from build123d import *


with BuildPart() as f1:
    # F0 (on Front) → F1 (revolve)
    with BuildSketch(Plane.XZ):
        Polygon((0, 8), (0, 0), (4, 0), (4, 8.25), (4, 9), (0, 9), align=None)
        Polygon((4, 9), (4, 8.25), (6, 8.25), (6, 11), (4, 11), align=None)
    revolve(axis=Axis((0, 0, 4), (0, 0, 1)))


solid = f1.part
Check sheet for the modelled part. Datum: model origin and axes. Units: mm. A direction names the side the tool comes from. Round coordinates to 2 decimals unless told otherwise and drop trailing zeros. Order: outer loops, then holes, each group sorted by start corner. A loop starts at its lowest first (then second) coordinate and runs counter-clockwise, first axis right, second up.
(1) Access from +Z, -Z, +X, -X, +Y, -Y to the whole of each face (thin tool, end or side, straight path). Record for faces 1 (the flat face through (0, 0, 0)), 2 (the flat face through (1.42, -3.92, 8.25)), 3 (the flat face through (0, 0, 9)).
(2) Go/stop test with flat-tipped pins: P1, Ø2, axis at x = 0, z = 4, coming from the +Y side; P2, Ø3, axis at y = -4.5, z = 5.5, coming from the +X side; P3, Ø2.5, axis at x = 0, y = -1, coming from the +Z side. Record where each tip stops, or that it passes through.
(3) Scan lines: probe 1 along Y at (x, z) = (0, 10.15); probe 2 along Z at (x, y) = (-1.75, 5.5); probe 3 along Z at (x, y) = (1.25, 1.75). Record each from-to range of solid material in increasing order.
(4) Cross-section at C-C, the plane z = 9.75. Enter the section's corners in (x, y).
(5) Cross-section at A-A, the plane x = 0. Enter the section's corners in (y, z), and give its area (3 significant figures).
(6) Cross-section at D-D, the plane z = 5. Enter the section's corners in (x, y), and give its area (3 significant figures).
(7) Draft check along Y on faces 4 (the flat face through (-1.42, -3.92, 11)), 5 (the cylindrical face through (-0.867, -3.905, 4.183)), 6 (the cylindrical face through (-0.867, -3.905, 9.986)). Enter one of: pulls with the +Y half, pulls with the -Y half, needs draft (parallel to the pull), parting line crosses it, or undercut.
Check sheet entries:
1. face 1: -Z, +X, -X, +Y, -Y
1. face 2: -Z
1. face 3: +Z
2. P1: stops at y = 4
2. P2: stops at x = 2.65
2. P3: stops at z = 9
3. probe 1: y = -6 to -4, 4 to 6
3. probe 2: z = 8.25 to 11
3. probe 3: z = 0 to 9
4. outline: circle Ø12 at (0, 0); hole circle Ø8 at (0, 0)
5. outline: (-6, 8.25) - (-4, 8.25) - (-4, 0) - (4, 0) - (4, 8.25) - (6, 8.25) - (6, 11) - (4, 11) - (4, 9) - (-4, 9) - (-4, 11) - (-6, 11) - close
5. area: 83.0 mm2
6. outline: circle Ø8 at (0, 0)
6. area: 50.3 mm2
7. face 4: needs draft
7. face 5: parting line crosses it
7. face 6: undercut
